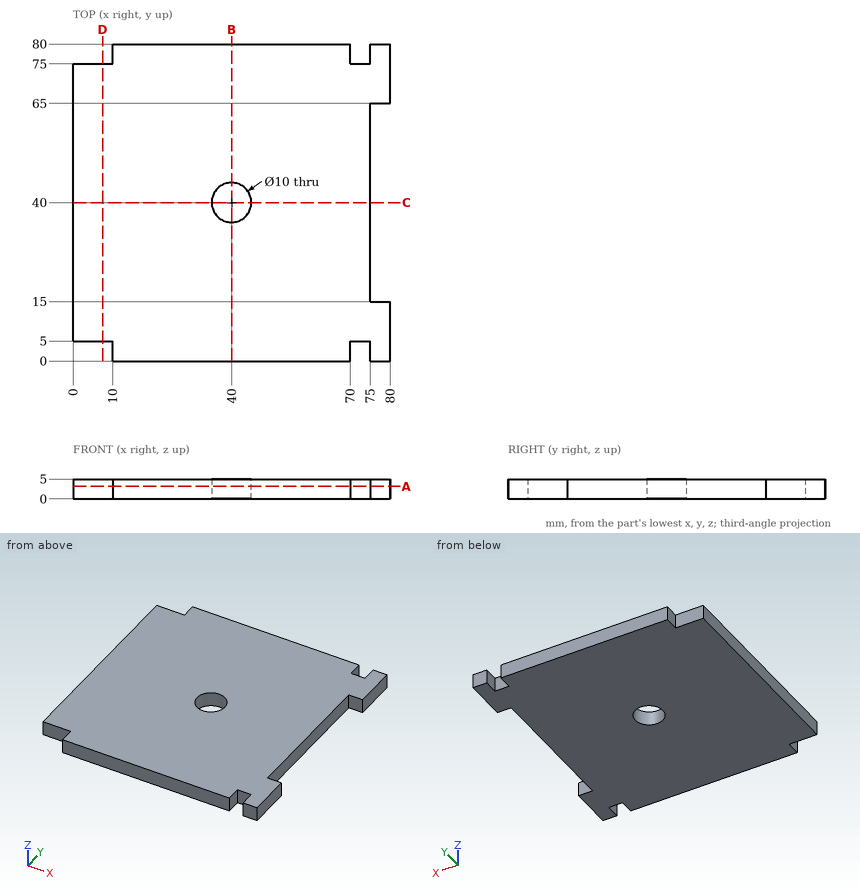
Job drawing, mm, ordinate dimensions from the low corner. One solid piece. Give positions to 0.01 mm unless a question says otherwise; leave off trailing zeros. Order: outer loops, then holes, each group sorted by start corner. A loop starts at its lowest first (then second) coordinate and runs counter-clockwise, first axis right, second up. Notation, with made-up numbers: (31, 16.5) -> (55, 16.5) arc R28 ccw to (55, 41.5) -> close; hole circle Ø5 at (55.5, 18). An arc over 180 degrees is marked (long way). Return JSON: item names as keys, results as strings.
Q1. Flat gauge pins, fed straight in: pin 1 (8 mm diameter, centred on x = 40, y = 40, fed in from +Z); pin 2 (6 mm diameter, centred on x = 20.5, y = 10, fed in from -Z); pin 3 (1.5 mm diameter, centred on x = 73.5, z = 3, fed in from +Y); pin 4 (1.5 mm diameter, centred on y = 2, z = 2.5, fed in from -X). Where does each tip first touch, or does it go through?
Working result:
{"pin 1": "through", "pin 2": "z = 0", "pin 3": "y = 75", "pin 4": "x = 10"}
Q2. Saw through at C-C (y = 40). Write the cut outline in (x, z).
Working result:
{"outline": "(0, 0) -> (35, 0) -> (35, 5) -> (0, 5) -> close; (45, 0) -> (75, 0) -> (75, 5) -> (45, 5) -> close"}
Q3. Saw through at A-A (z = 3.15). Write the cut outline in (x, y).
Working result:
{"outline": "(0, 5) -> (10, 5) -> (10, 0) -> (70, 0) -> (70, 5) -> (75, 5) -> (75, 0) -> (80, 0) -> (80, 15) -> (75, 15) -> (75, 65) -> (80, 65) -> (80, 80) -> (75, 80) -> (75, 75) -> (70, 75) -> (70, 80) -> (10, 80) -> (10, 75) -> (0, 75) -> close; hole circle Ø10 at (40, 40)"}
Q4. Drill centre lines: line 1 (Y direction, x = 40, z = 3.7); line 2 (Y direction, x = 76.5, z = 2.1); line 3 (X direction, y = 46, z = 1.55). Where is each one in solid material? Low to high.
Working result:
{"line 1": "0 to 35, 45 to 80", "line 2": "0 to 15, 65 to 80", "line 3": "0 to 75"}
Q5. Saw through at D-D (x = 7.5). Write the cut outline in (y, z).
Working result:
{"outline": "(5, 0) -> (75, 0) -> (75, 5) -> (5, 5) -> close"}
Q6. Saw through at B-B (x = 40). Write the cut outline in (y, z).
Working result:
{"outline": "(0, 0) -> (35, 0) -> (35, 5) -> (0, 5) -> close; (45, 0) -> (80, 0) -> (80, 5) -> (45, 5) -> close"}
